Design review of the part shown in the three views and the two pictorial views. Dimensions are in mm from the part's minimum x, y and z. Round coordinates to 2 decimals unless told otherwise and drop trailing zeros. Loops run counter-clockwise (first coordinate to the right, second up) from the corner with the lowest first, then second, coordinate; pieces in that order, holes last. Notation, with made-up numbers: (78, 5.5) -> (116, 5.5) arc R28 cw to (116, 23.5) -> close; hole circle Ø8 at (-13.75, 89). An arc over 180 degrees is marked (long way). Use a Markdown table: item, result. Add a question column.
1) Consider section C-C on y = 1.65. Give the boundary of the cut face in (x, z).
2) Insertion check: pin 1 (7 mm diameter, centred on x = 53, z = 7.5, fed in from -Y). The pin has a flat end and moves straight along its axis. Give the tip position at first contact, or say it passes through.
3) Consider section A-A on x = 53. Give the boundary of the cut face in (y, z), plus the area to 3 significant figures.
4) Wall thickness on probe 1 along X at (y, z) = (1.1, 7.5); probe 2 along X at (y, z) = (1, 6); probe 3 along Z at (x, y) = (55.5, 1.9): over which ranges is each line inside the solid? List them lowest first.
5) Consider section B-B on z = 7.5. Give the boundary of the cut face in (x, y).
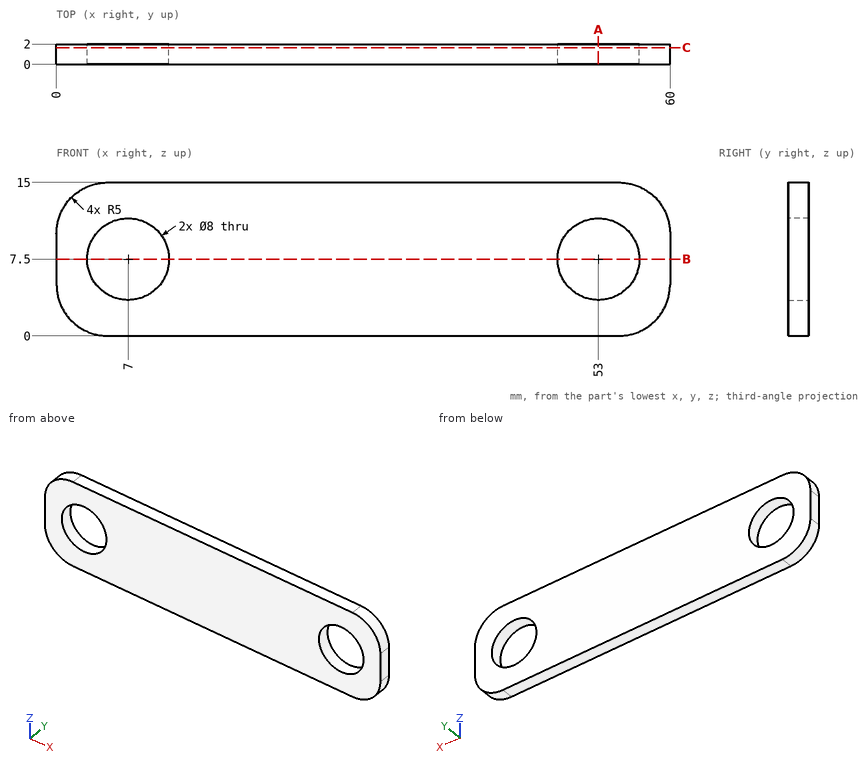
Result set:
| question | item | result |
|---|---|---|
| 1 | outline | (0, 5) arc R5 ccw to (5, 0) -> (55, 0) arc R5 ccw to (60, 5) -> (60, 10) arc R5 ccw to (55, 15) -> (5, 15) arc R5 ccw to (0, 10) -> close; hole circle Ø8 at (7, 7.5); hole circle Ø8 at (53, 7.5) |
| 2 | pin 1 | through |
| 3 | outline | (0, 0) -> (2, 0) -> (2, 3.5) -> (0, 3.5) -> close; (0, 11.5) -> (2, 11.5) -> (2, 15) -> (0, 15) -> close |
| 3 | area | 14.0 mm2 |
| 4 | probe 1 | 0 to 3, 11 to 49, 57 to 60 |
| 4 | probe 2 | 0 to 3.29, 10.71 to 49.29, 56.71 to 60 |
| 4 | probe 3 | 0.03 to 4.38, 10.62 to 14.97 |
| 5 | outline | (0, 0) -> (3, 0) -> (3, 2) -> (0, 2) -> close; (11, 0) -> (49, 0) -> (49, 2) -> (11, 2) -> close; (57, 0) -> (60, 0) -> (60, 2) -> (57, 2) -> close |
